Part print with two shaded views. Sizes in mm from the minimum x, y, z corner. A direction names the side the tool comes from. Round coordinates to 2 decimals unless told otherwise and drop trailing zeros. Write each loop counter-clockwise with the first axis right and the second up, starting at its lowest first coordinate (ties: lowest second). Pieces come first, ordered by that corner, then holes. Notation, with made-up numbers: (16.5, 68) -> (71.5, 68) arc R20 cw to (71.5, 83) -> close; hole circle Ø3 at (47, 0). An arc over 180 degrees is marked (long way). Return JSON: item names as keys, results as strings. Group by question number.
(1) Saw through at D-D (y = 38). List the corners of the cut face in (x, z).
(2) Saw through at C-C (x = 23.5). List the corners of the cut face in (y, z), plus the area to 3 significant figures.
(3) Drill centre lines: L1, parallel to Z at x = 51.5, y = 1.6; L2, parallel to Z at x = 24, y = 11.5; L3, parallel to Y at x = 60.5, z = 6.5. Where is each one in solid material? Low to high. Write a range as from..to.
(4) Saw through at B-B (z = 10). List the corners of the cut face in (x, y), plus the area to 3 significant figures.
(5) Drop flat-ended pins along their axis: pin 1 Ø6 at (x, z) = (20, 5.5) entering from +Y; pin 2 Ø5 at (x, y) = (7.5, 13) entering from -Z; pin 3 Ø2.5 at (x, z) = (11.5, 10) entering from -Y. Give the stop position or say it passes through.
(6) Saw through at A-A (x = 51.5). List the corners of the cut face in (y, z).
(7) Tool access for the marked faces 1 and 2: list every direction of +Z, -Z, +X, -X, +Y, -Y with a clear straight run to the whole face (end or side of a thin tool).
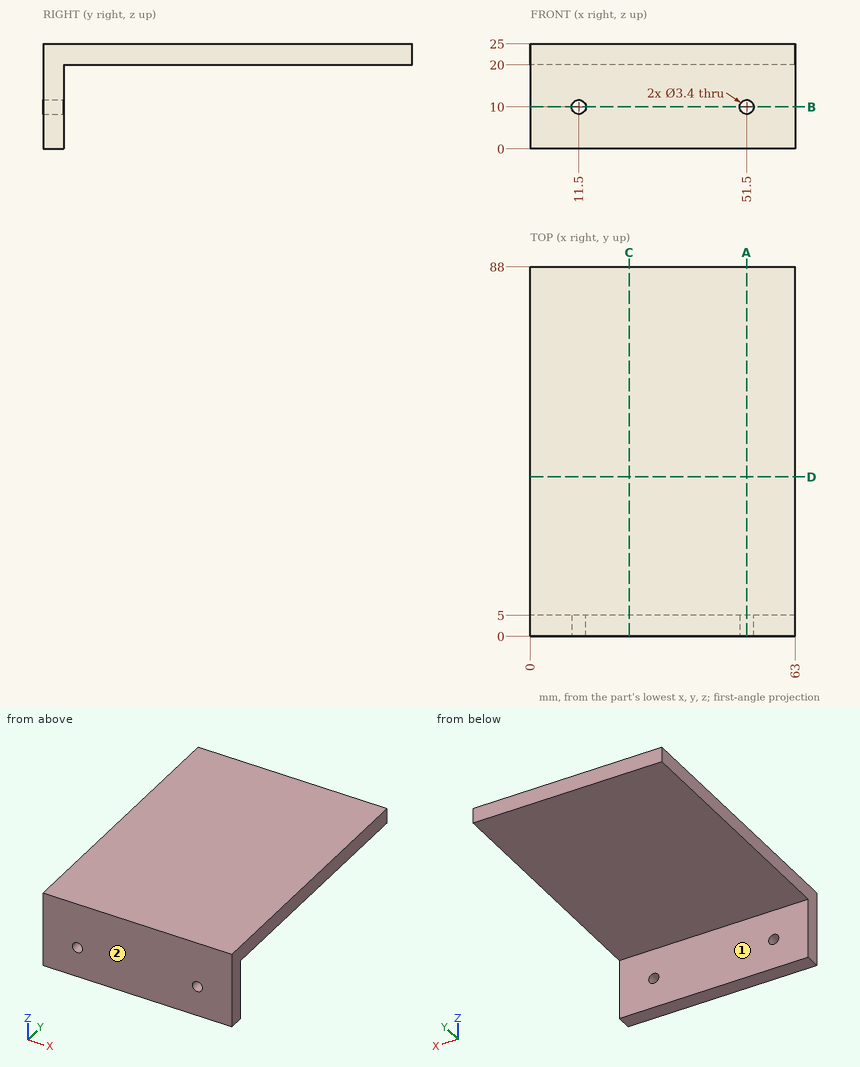
Computed values:
{
 "1": {"outline": "(0, 20) -> (63, 20) -> (63, 25) -> (0, 25) -> close"},
 "2": {"outline": "(0, 0) -> (5, 0) -> (5, 20) -> (88, 20) -> (88, 25) -> (0, 25) -> close", "area": "540 mm2"},
 "3": {"L1": "0..8.3, 11.7..25", "L2": "20..25", "L3": "0..5"},
 "4": {"outline": "(0, 0) -> (9.8, 0) -> (9.8, 5) -> (0, 5) -> close; (13.2, 0) -> (49.8, 0) -> (49.8, 5) -> (13.2, 5) -> close; (53.2, 0) -> (63, 0) -> (63, 5) -> (53.2, 5) -> close", "area": "281 mm2"},
 "5": {"pin 1": "y = 5", "pin 2": "z = 20", "pin 3": "through"},
 "6": {"outline": "(0, 0) -> (5, 0) -> (5, 8.3) -> (0, 8.3) -> close; (0, 11.7) -> (5, 11.7) -> (5, 20) -> (88, 20) -> (88, 25) -> (0, 25) -> close"},
 "7": {"face 1": "-Z, +X, -X, +Y", "face 2": "+Z, -Z, +X, -X, -Y"}
}
